Geometry check sheet. Reference: drawing and pictorial views, mm from the part's lowest x, y, z. Give positions to 0.01 mm unless a question says otherwise; leave off trailing zeros. Loops run counter-clockwise (first coordinate to the right, second up) from the corner with the lowest first, then second, coordinate; pieces in that order, holes last. Notation, with made-up numbers: (16, -22.5) -> (57, -22.5) arc R31 cw to (57, 16.5) -> close; hole circle Ø5 at (-23.75, 64). An arc over 180 degrees is marked (long way). One line per item, written item: value. Start each with the question number.
(1) Scan lines: line 1 along Z through (x, y) = (497, 4.5); line 2 along X through (y, z) = (11.75, 390.5). Record each from-to range of solid material in increasing order. Write a range as from..to.
(2) Sectioned sample at A-A, the plane x = 125.5. Record the cut outline in (y, z).
(3) Sectioned sample at C-C, the plane z = 477. Record the cut outline in (x, y).
(4) Sectioned sample at B-B, the plane y = 13.5. Record the cut outline in (x, z).
(5) Gauge pin test, flat end, axial feed: pin 1 Ø10 at (y, z) = (11.5, 406.5) entering from +X. Record the tip position at first contact, or that the pin passes through.
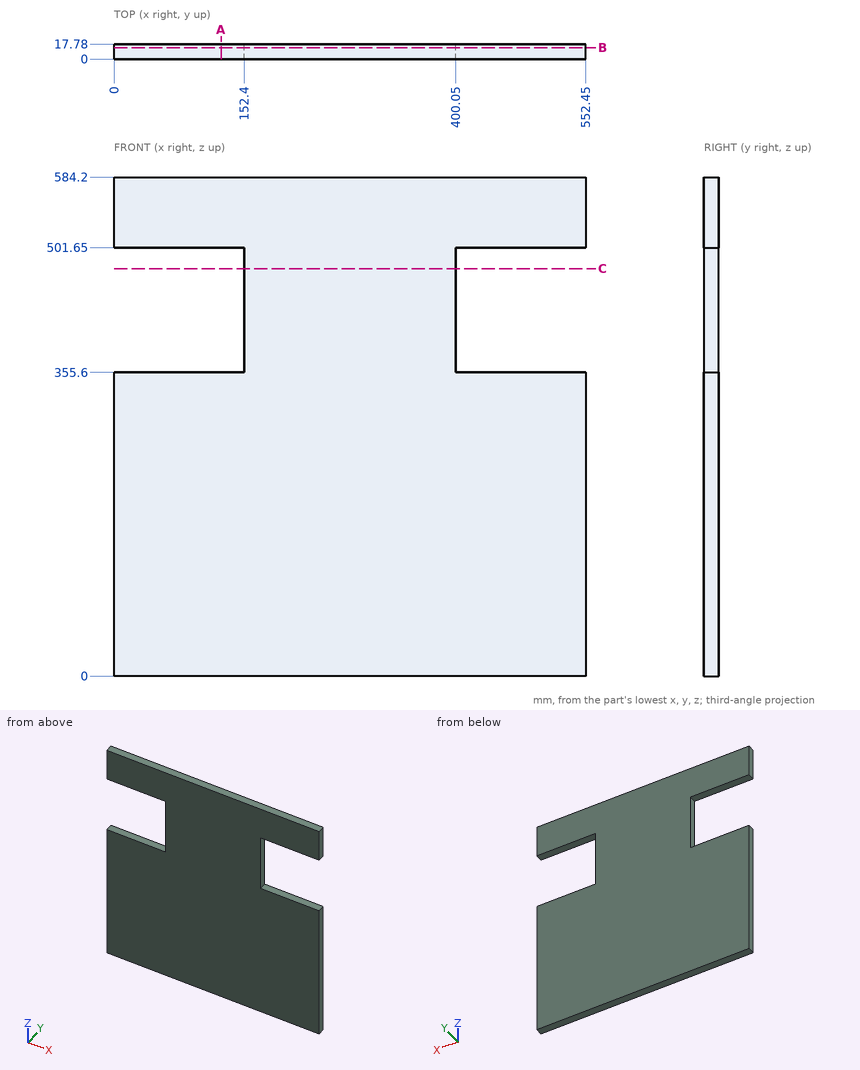
Calculated:
1. line 1: z = 0..355.6, 501.65..584.2
1. line 2: x = 152.4..400.05
2. outline: (0, 0) -> (17.78, 0) -> (17.78, 355.6) -> (0, 355.6) -> close; (0, 501.65) -> (17.78, 501.65) -> (17.78, 584.2) -> (0, 584.2) -> close
3. outline: (152.4, 0) -> (400.05, 0) -> (400.05, 17.78) -> (152.4, 17.78) -> close
4. outline: (0, 0) -> (552.45, 0) -> (552.45, 355.6) -> (400.05, 355.6) -> (400.05, 501.65) -> (552.45, 501.65) -> (552.45, 584.2) -> (0, 584.2) -> (0, 501.65) -> (152.4, 501.65) -> (152.4, 355.6) -> (0, 355.6) -> close
5. pin 1: stops at x = 400.05
